from build123d import *

# Parameters (mm, degrees)
F2_SIZE = 0.762
F3_SIZE = 5.08
F4_R    = 13.97


with BuildPart() as f1:
    # F0 (on Front) → F1 (revolve)
    with BuildSketch(Plane.XZ):
        Polygon((-9.65059, 57.969252), (-43.776404, 57.969252), (-43.776404, 23.401398), (38.797457, 23.401398), (38.797457, 43.823838), (21.999775, 43.823838), (21.999775, 39.226579), (9.799354, 39.226579), (9.799354, 43.823838), (-9.65059, 43.823838), align=None)
    revolve(axis=Axis((-2.489474, 0, 0), (1, 0, 0)))

    # F2
    f2_edges = [f1.edges().sort_by_distance(p)[0] for p in [
        (38.797457, 0, -43.823838),
        (21.999775, 0, -43.823838),
        (9.799354, 0, -43.823838),
        (9.799354, 0, -39.226579),
        (21.999775, 0, -39.226579),
    ]]
    chamfer(f2_edges, length=F2_SIZE)

    # F3
    f3_edges = [f1.edges().sort_by_distance(p)[0] for p in [
        (38.797457, 0, -23.401398),
    ]]
    chamfer(f3_edges, length=F3_SIZE)

    # F4
    f4_edges = [f1.edges().sort_by_distance(p)[0] for p in [
        (-9.65059, 0, -43.823838),
    ]]
    fillet(f4_edges, radius=F4_R)


solid = f1.part
Input: part model. Units: mm. Frame: model coordinates. A direction names the side the tool comes from. Give positions to 0.01 mm unless a question says otherwise; leave off trailing zeros. Order: outer loops, then holes, each group sorted by start corner. A loop starts at its lowest first (then second) coordinate and runs counter-clockwise, first axis right, second up. Notation, with made-up numbers: M -32,1.5 L -25,1.5 A25 ccw -25,21.5 Z; hole C 59.5,22 d11. An arc over 180 degrees is marked long. Answer as a JSON object with one key per item and string values.
1. Ray query, line 1 (Z direction, x = 12, y = 0); line 2 (Z direction, x = -22, y = 0); line 3 (Y direction, x = 6, z = 0). Return the intervals inside material, ascending. Write a range as [from, to].
Result sheet:
{"line 1": "[-39.23, -23.4], [23.4, 39.23]", "line 2": "[-57.97, -23.4], [23.4, 57.97]", "line 3": "[-43.82, -23.4], [23.4, 43.82]"}
2. Cut plane C-C, the plane x = -36. Output: boundary loops of the cut face in (y, z), and give its area (3 significant figures).
Result sheet:
{"outline": "C 0,0 d115.94; hole C 0,0 d46.8", "area": "8,840 mm²"}
3. Reachability of faces 4 (the flat face through (22, 38, 13)), 5 (the cylindrical face through (30.292, 26.666, -34.777)), 6 (the cylindrical face through (-26.952, -17.412, 55.292)) from +Z, -Z, +X, -X, +Y, -Y: full face, straight path, thin tool, end or side. Return the list, or none.
Result sheet:
{"face 4": "none", "face 5": "+X", "face 6": "+X, -X"}
4. Pull-direction query (X, two-part tool) for faces 1 (the flat face through (-43.776, -1, 25)), 2 (the cylindrical face through (6.645, 26.666, -34.777)), 3 (the cylindrical face through (15.82, -26.51, -28.91)); classes: +X half, -X half, draft (parallel to the pull), parting line (faces both ways), or undercut.
Result sheet:
{"face 1": "-X half", "face 2": "draft", "face 3": "undercut"}
5. Cut plane D-D, the plane x = 0.5. Output: boundary loops of the cut face in (y, z).
Result sheet:
{"outline": "C 0,0 d88.71; hole C 0,0 d46.8"}
6. First-contact query: P1, Ø1.5, axis at y = -5.5, z = 20, coming from the +X side; P2, Ø5, axis at x = 11.5, y = 28.5, coming from the +Z side; P3, Ø3, axis at x = 4, z = 10.5, coming from the -Y side; P4, Ø2, axis at y = 40, z = -33, coming from the +X side. Flat tips, straight axial feed; report the tip coordinate or a pass-through.
Result sheet:
{"P1": "through", "P2": "z = 33.94", "P3": "y = -42.9", "P4": "x = -7.81"}
